For this review, take the finished solid that the model builds, in its own axes (mm). A direction names the side the tool comes from. Give positions to 0.01 mm unless a question says otherwise; leave off trailing zeros. Write each loop counter-clockwise with the first axis right and the second up, starting at its lowest first coordinate (ties: lowest second). Pieces come first, ordered by that corner, then holes.
1) Machinability: for faces 1 (the face through (1192.386, -426, -401)), 2 (the face through (688, 315.303, -401)), 3 (the face through (501, 35.903, -401)), which of the approach directions +Z, -Z, +X, -X, +Y, -Y give a long, thin tool a straight path to every point of the face, cutting with its end or side? Answer none if there is none.
2) We need section C-C on x = 100.5. Give the boundary of the cut face in (y, z).
3) Wall thickness on line 1 along Y through (x, z) = (736, -409.5); line 2 along X through (y, z) = (94, -406); line 3 along X through (y, z) = (-97, -283): over which ranges is each line inside the solid? List them lowest first.
4) For P1, Ø12, axis at y = -49, z = -179.5, coming from the +X side; P2, Ø12, axis at y = 86.5, z = -582, coming from the -X side; P3, Ø2, axis at y = -175, z = -460.5, coming from the -X side, all flat-tipped, find the tip position at first contact; note any pin that passes through.
5) We need section A-A on y = -637. Give the boundary of the cut face in (x, z), and give its area (3 significant figures).
6) We need section D-D on z = -689. Give the boundary of the cut face in (x, y), and give its area (3 significant figures).
7) We need section B-B on z = -544. Give the boundary of the cut face in (x, y).
8) Draft analysis for pull direction X (two halves, no side actions). For faces 4 (the face through (2005.186, -196, -403)), 5 (the face through (515, -421.297, -401)), 6 (the face through (912.986, -189, -401)), 7 (the face through (465.7, 173.6, -484.2)), state which applies: pulls with the +X half, pulls with the -X half, needs draft (parallel to the pull), parting line crosses it, or undercut.
from build123d import *

# Parameters (mm, degrees)
F1_DEPTH = 812.8
F2_W     = 812.8
F2_H     = 177.8
F3_DEPTH = 736.601
F4_R     = 203.2
F5_DEPTH = 1016.001
F7_DEPTH = 812.8


with BuildPart() as f1:
    # F0 (on Top) → F1 (new body)
    with BuildSketch(Plane.XY):
        Polygon((1192.385533, 315.303055), (-128.414467, 315.303055), (-128.414467, 35.903055), (912.985533, 35.903055), (912.985533, -421.296945), (-128.414467, -421.296945), (-128.414467, -700.696945), (1192.385533, -700.696945), (1192.385533, -421.296945), (2005.185533, -421.296945), (2005.185533, 35.903055), (1192.385533, 35.903055), align=None)
    extrude(amount=-F1_DEPTH)

    # F2 (on face) → F3 (cut, through all)
    with BuildSketch(Plane.XZ.offset(421.296945)):
        with Locations((1598.785533, -88.9)):
            Rectangle(F2_W, F2_H)
        with Locations((1598.785533, -723.9)):
            Rectangle(F2_W, F2_H)
    extrude(amount=-F3_DEPTH, mode=Mode.SUBTRACT)

    # F4 (on face) → F5 (cut, through all)
    with BuildSketch(Plane.XZ.offset(700.696945)):
        with BuildLine():
            ThreePointArc((-128.414467, -406.4), (-9.382663, -119.031804), (277.985533, 0))
            Line((277.985533, 0), (-128.414467, 0))
            Line((-128.414467, 0), (-128.414467, -406.4))
        make_face()
        with BuildLine():
            ThreePointArc((277.985533, -812.8), (-9.382663, -693.768196), (-128.414467, -406.4))
            Line((-128.414467, -406.4), (-128.414467, -812.8))
            Line((-128.414467, -812.8), (277.985533, -812.8))
        make_face()
        with Locations((277.985533, -406.4)):
            Circle(F4_R)
    extrude(amount=-F5_DEPTH, mode=Mode.SUBTRACT)

    # F6 (on face) → F7 (cut)
    with BuildSketch(Plane.YZ.offset(2005.185533)):
        with BuildLine():
            Line((-421.296945, -635), (-192.696945, -635))
            ThreePointArc((-192.696945, -635), (-354.341555, -568.04461), (-421.296945, -406.4))
            Line((-421.296945, -406.4), (-421.296945, -635))
        make_face()
        with BuildLine():
            Line((35.903055, -635), (35.903055, -406.4))
            ThreePointArc((35.903055, -406.4), (-31.052335, -568.04461), (-192.696945, -635))
            Line((-192.696945, -635), (35.903055, -635))
        make_face()
        with BuildLine():
            ThreePointArc((-421.296945, -406.4), (-354.341555, -244.75539), (-192.696945, -177.8))
            Line((-192.696945, -177.8), (-421.296945, -177.8))
            Line((-421.296945, -177.8), (-421.296945, -406.4))
        make_face()
        with BuildLine():
            ThreePointArc((-192.696945, -177.8), (-31.052335, -244.75539), (35.903055, -406.4))
            Line((35.903055, -406.4), (35.903055, -177.8))
            Line((35.903055, -177.8), (-192.696945, -177.8))
        make_face()
    extrude(amount=-F7_DEPTH, mode=Mode.SUBTRACT)


solid = f1.part
Results list:
1. face 1: +X
1. face 2: +Z, -Z, +X, -X, +Y
1. face 3: +Z, -Z, -X
2. outline: (-700.7, -772) - (-421.3, -772) - (-421.3, -505.34) - (-700.7, -505.34) - close; (-700.7, -307.46) - (-421.3, -307.46) - (-421.3, -40.8) - (-700.7, -40.8) - close; (35.9, -772) - (315.3, -772) - (315.3, -505.34) - (35.9, -505.34) - close; (35.9, -307.46) - (315.3, -307.46) - (315.3, -40.8) - (35.9, -40.8) - close
3. line 1: y = -700.7 to -421.3, 35.9 to 315.3
3. line 2: x = -128.41 to 74.79, 481.19 to 1192.39
3. line 3: x = 912.99 to 2005.19
4. P1: stops at x = 1192.39
4. P2: stops at x = -91.33
4. P3: stops at x = 912.99
5. outline: (277.99, -812.8) - (1192.39, -812.8) - (1192.39, 0) - (277.99, 0) arc R406.4 ccw to start; hole circle Ø406.4 at (277.99, -406.4)
5. area: 873,000 mm2
6. outline: (-14.07, -700.7) - (1192.39, -700.7) - (1192.39, 315.3) - (-14.07, 315.3) - (-14.07, 35.9) - (912.99, 35.9) - (912.99, -421.3) - (-14.07, -421.3) - close
6. area: 802,000 mm2
7. outline: (-104.41, -700.7) - (128.46, -700.7) - (128.46, -421.3) - (-104.41, -421.3) - close; (-104.41, 35.9) - (128.46, 35.9) - (128.46, 315.3) - (-104.41, 315.3) - close; (427.51, -700.7) - (1192.39, -700.7) - (1192.39, -375.25) - (2005.19, -375.25) - (2005.19, -10.15) - (1192.39, -10.15) - (1192.39, 315.3) - (427.51, 315.3) - (427.51, 35.9) - (912.99, 35.9) - (912.99, -421.3) - (427.51, -421.3) - close
8. face 4: pulls with the +X half
8. face 5: needs draft
8. face 6: pulls with the -X half
8. face 7: undercut
